Design review of the part built by this model. Coordinates are the model's own, in mm. A direction names the side the tool comes from. Give positions to 0.01 mm unless a question says otherwise; leave off trailing zeros. Order: outer loops, then holes, each group sorted by start corner. A loop starts at its lowest first (then second) coordinate and runs counter-clockwise, first axis right, second up. Notation, with made-up numbers: M 68,39.5 L 120,39.5 A22 ccw 120,58.5 Z; hole C -14.75,26 d8. An arc over 180 degrees is marked long. Answer as a JSON object with one key per item and string values.
from build123d import *

# Parameters (mm, degrees)
BOSS_EXTRUDE1_START     = -3
BOSS_EXTRUDE1_OUTLINE_R = 1.5
BOSS_EXTRUDE1_DEPTH     = 3
SCALE1_SCALE            = 1.9


# Read off the part's stored shape, not the designer's step: Boss-Extrude1
with BuildPart() as part:
    # Boss-Extrude1 outline → Boss-Extrude1 (new body)
    with BuildSketch(Plane.XY.offset(BOSS_EXTRUDE1_START)):
        with BuildLine():
            Line((11.834550238, -2.472148997), (31.252104769, 0.084220555))
            ThreePointArc((31.252104769, 0.084220555), (34.695779445, 4.572104769), (30.207895231, 8.015779445))
            Line((30.207895231, 8.015779445), (13.427938823, 5.806656275))
            ThreePointArc((13.427938823, 5.806656275), (13.410760304, 5.846221532), (13.393465207, 5.885735968))
            ThreePointArc((13.393465207, 5.885735968), (12.041551488, 5.897071585), (10.729192217, 5.572244952))
            Line((10.729192217, 5.572244952), (10.189200244, 6.507557022))
            ThreePointArc((10.189200244, 6.507557022), (11.126720661, 7.481723913), (11.792869471, 8.658240563))
            ThreePointArc((11.792869471, 8.658240563), (11.606759368, 8.906179706), (11.415437385, 9.150119633))
            ThreePointArc((11.415437385, 9.150119633), (10.106597569, 8.81117421), (8.922976471, 8.15773197))
            ThreePointArc((8.922976471, 8.15773197), (8.549706323, 8.548135574), (8.159371308, 8.921477448))
            ThreePointArc((8.159371308, 8.921477448), (8.812813548, 10.105098546), (9.151758972, 11.413938362))
            Line((9.151758972, 11.413938362), (8.659879901, 11.791370448))
            ThreePointArc((8.659879901, 11.791370448), (7.483516811, 11.125336137), (6.509436976, 10.187999326))
            ThreePointArc((6.509436976, 10.187999326), (6.047829045, 10.468613272), (5.574146563, 10.728326528))
            ThreePointArc((5.574146563, 10.728326528), (5.898805358, 12.040487702), (5.887415057, 13.392168338))
            Line((5.887415057, 13.392168338), (5.314609747, 13.629432066))
            ThreePointArc((5.314609747, 13.629432066), (4.351003751, 12.681995862), (3.65280527, 11.524977816))
            ThreePointArc((3.65280527, 11.524977816), (3.134170467, 11.676689406), (2.609274564, 11.805074597))
            ThreePointArc((2.609274564, 11.805074597), (2.58305967, 13.15599481), (2.222297371, 14.458117388))
            Line((2.222297371, 14.458117388), (1.607601557, 14.539043627))
            ThreePointArc((1.607601557, 14.539043627), (0.922327421, 13.375148622), (0.547316802, 12.077605074))
            ThreePointArc((0.547316802, 12.077605074), (0.006856042, 12.089998056), (-0.533618427, 12.078218055))
            ThreePointArc((-0.533618427, 12.078218055), (-0.908651119, 13.375486662), (-1.593822374, 14.539142845))
            Line((-1.593822374, 14.539142845), (-2.208518188, 14.458216606))
            ThreePointArc((-2.208518188, 14.458216606), (-2.569071942, 13.157522433), (-2.595800172, 11.808044777))
            ThreePointArc((-2.595800172, 11.808044777), (-3.121351418, 11.680122659), (-3.640655008, 11.528821757))
            ThreePointArc((-3.640655008, 11.528821757), (-4.338480819, 12.683812024), (-5.300881923, 13.629722958))
            Line((-5.300881923, 13.629722958), (-5.873687233, 13.39245923))
            ThreePointArc((-5.873687233, 13.39245923), (-5.885433032, 12.043808909), (-5.562611018, 10.734312212))
            ThreePointArc((-5.562611018, 10.734312212), (-6.037455135, 10.474599539), (-6.500199913, 10.193895285))
            ThreePointArc((-6.500199913, 10.193895285), (-7.47268922, 11.127885908), (-8.646251294, 11.791833189))
            Line((-8.646251294, 11.791833189), (-9.138130365, 11.414401103))
            ThreePointArc((-9.138130365, 11.414401103), (-8.80083054, 10.109699304), (-8.150983569, 8.92914144))
            ThreePointArc((-8.150983569, 8.92914144), (-8.542690029, 8.555147402), (-8.917254459, 8.163986338))
            ThreePointArc((-8.917254459, 8.163986338), (-10.097571821, 8.813551755), (-11.401949093, 9.15072269))
            Line((-11.401949093, 9.15072269), (-11.779381179, 8.658843619))
            ThreePointArc((-11.779381179, 8.658843619), (-11.116550367, 7.486781519), (-10.184349411, 6.515145975))
            ThreePointArc((-10.184349411, 6.515145975), (-10.46607819, 6.052215075), (-10.726778871, 5.577124264))
            ThreePointArc((-10.726778871, 5.577124264), (-12.034053776, 5.89841947), (-13.38017907, 5.886378776))
            Line((-13.38017907, 5.886378776), (-13.617442798, 5.313573465))
            ThreePointArc((-13.617442798, 5.313573465), (-12.674640857, 4.353631081), (-11.523783462, 3.656571444))
            ThreePointArc((-11.523783462, 3.656571444), (-11.67614775, 3.13618777), (-11.805025713, 2.60949572))
            ThreePointArc((-11.805025713, 2.60949572), (-13.149945407, 2.581153618), (-14.44612812, 2.221261089))
            Line((-14.44612812, 2.221261089), (-14.527054359, 1.606565275))
            ThreePointArc((-14.527054359, 1.606565275), (-13.368714152, 0.923687604), (-12.07756623, 0.548173302))
            ThreePointArc((-12.07756623, 0.548173302), (-12.089998597, 0.005825389), (-12.07808888, -0.536534252))
            ThreePointArc((-12.07808888, -0.536534252), (-13.369010177, -0.912066026), (-14.527153576, -1.594858655))
            Line((-14.527153576, -1.594858655), (-14.446227337, -2.20955447))
            ThreePointArc((-14.446227337, -2.20955447), (-13.151251636, -2.569269431), (-11.807551859, -2.598041398))
            ThreePointArc((-11.807551859, -2.598041398), (0.06437742, -12.089828599), (11.834550238, -2.472148997))
        make_face()
        with Locations((-7.5, 0)):
            Circle(BOSS_EXTRUDE1_OUTLINE_R, mode=Mode.SUBTRACT)
        Circle(BOSS_EXTRUDE1_OUTLINE_R, mode=Mode.SUBTRACT)
        with Locations((7.5, 0)):
            Circle(BOSS_EXTRUDE1_OUTLINE_R, mode=Mode.SUBTRACT)
        with Locations((30.73, 4.05)):
            Circle(BOSS_EXTRUDE1_OUTLINE_R, mode=Mode.SUBTRACT)
    extrude(amount=BOSS_EXTRUDE1_DEPTH)


with BuildPart() as part_1:
    # Scale1: scaled about (5.663998646, 1.349090427, -1.5)
    add(part.part.scale(SCALE1_SCALE).moved(Location((-5.097598781, -1.214181384, 1.35))))


solid = part_1.part
(1) Insertion check: pin 1 (2 mm diameter, centred on y = 17.5, z = -0.5, fed in from -X); pin 2 (1 mm diameter, centred on y = -12, z = 0.5, fed in from +X); pin 3 (1.5 mm diameter, centred on x = 30, z = -0.5, fed in from +Y). Each pin has a flat end and moves straight along its axis. Give the tip position at first contact, or say it passes through.
Checked values:
{"pin 1": "stops at x = -22", "pin 2": "stops at x = 15.44", "pin 3": "stops at y = 11.18"}
(2) Tool access review of faces 1 (the cylindrical face through (-28.07, -1.19, -1.54)), 2 (the cylindrical face through (-13.32, 22.86, -1.54)), 3 (the flat face through (35.576, -3.517, -1.54)), 4 (the cylindrical face through (-16.556, 18.695, -1.54)): name each direction out of +Z, -Z, +X, -X, +Y, -Y from which nothing blocks a thin tool from reaching the whole face with its end or side.
Checked values:
{"face 1": "+Z, -Z, -X", "face 2": "+Z, -Z, +Y", "face 3": "+Z, -Z, +X, -Y", "face 4": "+Z, -Z"}
(3) We need section C-C (x = 48.5). Write out the cut boundary in (y, z).
Checked values:
{"outline": "M -1.82,-4.35 L 13.52,-4.35 L 13.52,1.35 L -1.82,1.35 Z"}
(4) To check wall thickness, follow L1, parallel to X at y = 19, z = 0.8; L2, parallel to Y at x = -7, z = -0.3; L3, parallel to Y at x = 14.5, z = 0.45. State the ranges of each line that lie inside material, in increasing order. Write a range as from..to.
Checked values:
{"L1": "x = -22.16..-18.21, -16.01..5.81, 8.05..11.99", "L2": "y = -24.11..-3.34, 0.91..24.59", "L3": "y = -13.2..10.74, 11.35..15.68"}
(5) We need section A-A (z = -2.5). Count the separate pieces of the cut face and the enclosed holes in it, plus the area to 3 significant figures.
Checked values:
{"separate pieces": "1", "enclosed holes": "4", "area": "2,360 mm^2"}
(6) We need section B-B (y = -14). Write out the cut boundary in (x, z), plus the area to 3 significant figures.
Checked values:
{"outline": "M -24.18,-4.35 L 13.99,-4.35 L 13.99,1.35 L -24.18,1.35 Z", "area": "218 mm^2"}
